Geometry: final body of the model. Coordinates: model frame, mm. Give positions to 0.01 mm unless a question says otherwise; leave off trailing zeros. Answer in a Markdown table with one row per item. Add a question column.
1) Draft query along Z for faces 1 (the flat face through (-3, -20, 136)), 2 (the flat face through (-3, -40, 2)), 3 (the flat face through (-3, -20, -136)). Return one class per face: +Z half, -Z half, draft (parallel to the pull), parting line (faces both ways), or undercut.
2) Line query: line 1 (X direction, y = -3.75, z = 50); line 2 (Z direction, x = -50, y = -7). Output: solid intervals per line, ascending. Write a range as from..to.
3) First-contact query: P1, Ø2.5, axis at x = 50, z = -50, coming from the +Y side. Flat tip, straight axial feed; report the tip coordinate or a pass-through.
```python
from build123d import *

# Parameters (mm, degrees)
F0_W     = 440
F0_H     = 272
F1_DEPTH = 40
F2_D     = 4.4
F2_DEPTH = 10
F2_TIP   = 1.3218933619


with BuildPart() as f1:
    # F0 (on Front) → F1 (new body)
    with BuildSketch(Plane.XZ):
        Rectangle(F0_W, F0_H)
    extrude(amount=F1_DEPTH)

    # F2
    with Locations(Plane(origin=(0, 0, 0), x_dir=(1, 0, 0), z_dir=(0, 1, 0))):
        with Locations((50, -50), (-50, -50), (-50, 50), (50, 50)):
            Hole(F2_D / 2, depth=F2_DEPTH)
            with Locations((0, 0, -(F2_DEPTH + F2_TIP / 2))):  # 118° drill point
                Cone(0, F2_D / 2, F2_TIP, mode=Mode.SUBTRACT)


solid = f1.part
```
Evaluation:
| question | item | result |
|---|---|---|
| 1 | face 1 | +Z half |
| 1 | face 2 | draft |
| 1 | face 3 | -Z half |
| 2 | line 1 | -220..-52.2, -47.8..47.8, 52.2..220 |
| 2 | line 2 | -136..-52.2, -47.8..47.8, 52.2..136 |
| 3 | P1 | y = -10.57 |
